Geometry: final body of the model. Coordinates: model frame, mm. A direction names the side the tool comes from. Give positions to 0.01 mm unless a question says otherwise; leave off trailing zeros. Loops run counter-clockwise (first coordinate to the right, second up) from the corner with the lowest first, then second, coordinate; pieces in that order, holes last.
from build123d import *

# Parameters (mm, degrees)
SKETCH1_W               = 257.843094768
SKETCH1_H               = 107.95
BOSS_EXTRUDE1_DEPTH     = 6.35
SKETCH1_3_W             = 3.175
SKETCH1_3_H             = 90.678
BOSS_EXTRUDE2_DEPTH     = 19.05
SKETCH3_R               = 0.762
CUT_EXTRUDE1_DEPTH      = 6.35
SKETCH4_W               = 101.6
SKETCH4_H               = 101.6
CUT_EXTRUDE2_DEPTH      = 6.35
CUT_EXTRUDE3_DEPTH      = 20.574
CUT_EXTRUDE3_DEPTH_BACK = 86.614


with BuildPart() as part:
    # Sketch1 → Boss-Extrude1 (new body)
    with BuildSketch(Plane(origin=(0, 0, 0), x_dir=(1, 0, 0), z_dir=(0, 1, 0))):
        Rectangle(SKETCH1_W, SKETCH1_H)
    extrude(amount=-BOSS_EXTRUDE1_DEPTH)

    # Sketch1_3 → Boss-Extrude2 (add)
    with BuildSketch(Plane(origin=(0, 0, 0), x_dir=(1, 0, 0), z_dir=(0, 1, 0))):
        Polygon((-128.921547384, 53.975), (-128.921547384, 45.339), (-125.746547384, 45.339), (-122.571547384, 45.339), (-122.571547384, 53.975), align=None)
        Polygon((-96.917547384, 45.339), (-93.742547384, 45.339), (-93.742547384, 53.975), (-100.092547384, 53.975), (-100.092547384, 45.339), align=None)
        Polygon((-100.092547384, -45.339), (-100.092547384, -53.975), (-93.742547384, -53.975), (-93.742547384, -45.339), (-96.917547384, -45.339), align=None)
        Polygon((-128.921547384, -45.339), (-128.921547384, -53.975), (-122.571547384, -53.975), (-122.571547384, -45.339), (-125.746547384, -45.339), align=None)
        with Locations((-127.334047384, 0)):
            Rectangle(SKETCH1_3_W, SKETCH1_3_H)
        with Locations((-95.330047384, 0)):
            Rectangle(SKETCH1_3_W, SKETCH1_3_H)
    extrude(amount=BOSS_EXTRUDE2_DEPTH)

    # Sketch3 → Cut-Extrude1 (cut)
    with BuildSketch(Plane.XY.offset(53.975)):
        with Locations((-111.332047384, -1.651)):
            Circle(SKETCH3_R)
    cut_extrude1 = extrude(amount=-CUT_EXTRUDE1_DEPTH, mode=Mode.SUBTRACT)

    # Mirror1: Cut-Extrude1 across plane
    add(cut_extrude1.mirror(Plane.XY), mode=Mode.SUBTRACT)

    # Sketch4 → Cut-Extrude2 (cut)
    with BuildSketch(Plane(origin=(0, 0, 0), x_dir=(1, 0, 0), z_dir=(0, 1, 0))):
        with Locations((-33.003452616, 0)):
            Rectangle(SKETCH4_W, SKETCH4_H)
    extrude(amount=-CUT_EXTRUDE2_DEPTH, mode=Mode.SUBTRACT)

    # Sketch5 → Cut-Extrude3 (cut, two sides)
    with BuildSketch(Plane(origin=(0, 0, 0), x_dir=(1, 0, 0), z_dir=(0, 1, 0))) as cut_extrude3_sk:
        Polygon((-33.003452616, 81.208415926), (-33.003452616, 50.8), (-33.003452616, -61.928851746), (144.325230391, -61.928851746), (144.325230391, 81.208415926), align=None)
    extrude(amount=CUT_EXTRUDE3_DEPTH, mode=Mode.SUBTRACT)
    extrude(cut_extrude3_sk.sketch, amount=-CUT_EXTRUDE3_DEPTH_BACK, mode=Mode.SUBTRACT)


solid = part.part
Item 1: Set-up query: faces 4 (the face through (-124, 9, 45.339)), 5 (the face through (-93.743, 9, 1)), 6 (the face through (-83.803, -3, 1)), 7 (the face through (-122.572, 9, 50)). Return all of +Z, -Z, +X, -X, +Y, -Y with unobstructed straight access to the full face (end or side cutting, diameter ignored); none if empty.
Values follow:
face 4: +Y
face 5: +Z, -Z, +X, +Y
face 6: +X, +Y, -Y
face 7: +Z, -Z, +Y
Item 2: Section query C-C on z = 30.5. Return loops of the section in (x, y), plus the area to 3 significant figures.
Values follow:
outline: (-128.92, -6.35) - (-83.8, -6.35) - (-83.8, 0) - (-93.74, 0) - (-93.74, 19.05) - (-96.92, 19.05) - (-96.92, 0) - (-125.75, 0) - (-125.75, 19.05) - (-128.92, 19.05) - close
area: 407 mm2
Item 3: Section query A-A on y = 12.25. Return loops of the section in (x, z) (3 decimals).
Values follow:
outline: (-128.922, -53.975) - (-122.572, -53.975) - (-122.572, -45.339) - (-125.747, -45.339) - (-125.747, 45.339) - (-122.572, 45.339) - (-122.572, 53.975) - (-128.922, 53.975) - close; (-100.093, -53.975) - (-93.743, -53.975) - (-93.743, 53.975) - (-100.093, 53.975) - (-100.093, 45.339) - (-96.918, 45.339) - (-96.918, -45.339) - (-100.093, -45.339) - close
Item 4: Section query B-B on x = -56. Return loops of the section in (y, z) (3 decimals).
Values follow:
outline: (-6.35, -53.975) - (0, -53.975) - (0, -50.8) - (-6.35, -50.8) - close; (-6.35, 50.8) - (0, 50.8) - (0, 53.975) - (-6.35, 53.975) - close
Item 5: Ray query, probe 1 along Z at (x, y) = (-83.5, -0.75) (3 decimals); probe 2 along X at (y, z) = (7, -26); probe 3 along X at (y, z) = (3, 48.5). Return the intervals inside material, ascending.
Values follow:
probe 1: z = -53.975 to -50.8, 50.8 to 53.975
probe 2: x = -128.92 to -125.75, -96.92 to -93.74
probe 3: x = -128.92 to -122.57, -100.09 to -93.74
Item 6: Pin query (flat end, axial travel): pin 1 (14.5 mm diameter, centred on x = -110, z = -25.5, fed in from +Y); pin 2 (9.5 mm diameter, centred on y = 6, z = 17, fed in from +X); pin 3 (0.5 mm diameter, centred on x = -111, y = -1.5, fed in from -Z) (3 decimals). Return the tip coordinate at first contact, or that it passes through.
Values follow:
pin 1: stops at y = 0
pin 2: stops at x = -93.74
pin 3: stops at z = -47.625
Item 7: Draft query along Z for faces 1 (the face through (-86, 0, 0)), 2 (the face through (-91.8, -0.3, 53.975)), 3 (the face through (-59, -3, 50.8)). Return one class per face: +Z half, -Z half, draft (parallel to the pull), parting line (faces both ways), or undercut.
Values follow:
face 1: draft
face 2: +Z half
face 3: undercut
Item 8: Section query D-D on y = -4. Return loops of the section in (x, z) (3 decimals), plus the area to 3 significant figures.
Values follow:
outline: (-128.922, -53.975) - (-33.003, -53.975) - (-33.003, -50.8) - (-83.803, -50.8) - (-83.803, 50.8) - (-33.003, 50.8) - (-33.003, 53.975) - (-128.922, 53.975) - close
area: 5,190 mm2
